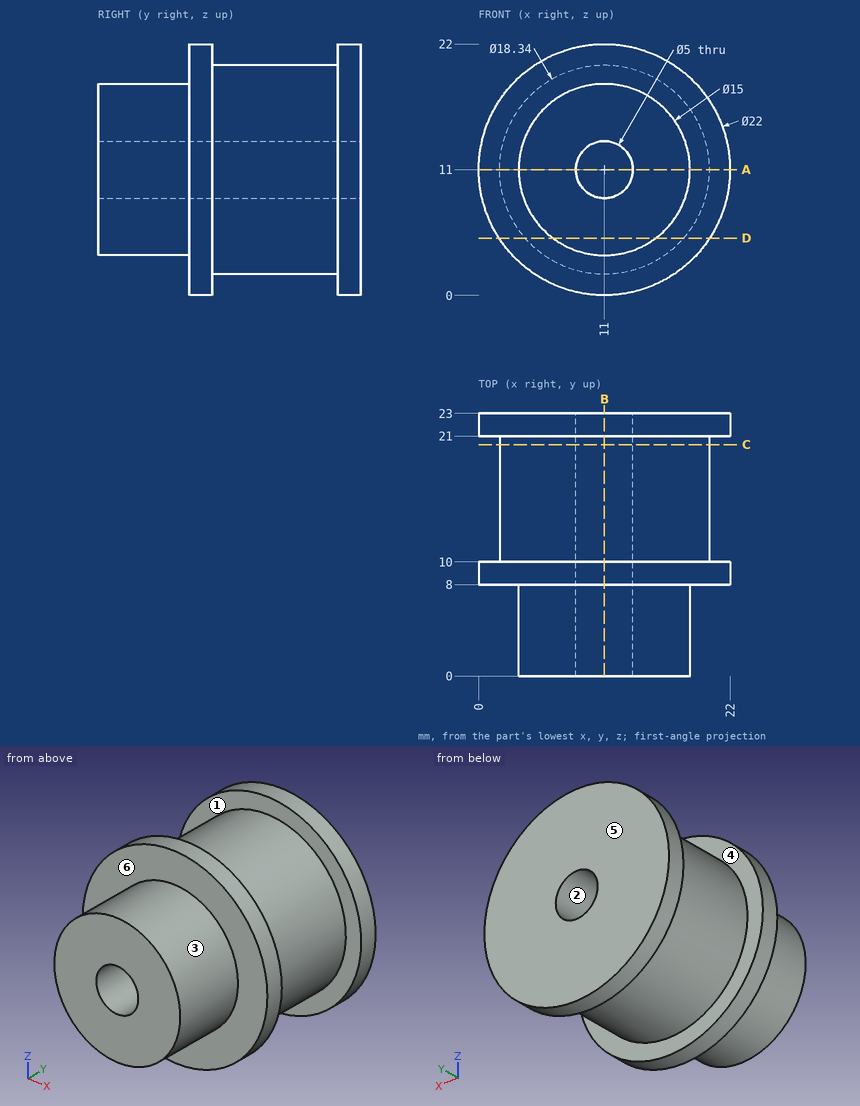
Check sheet for the drawn part. Datum: minimum x, y, z corner. Units: mm. A direction names the side the tool comes from. Round coordinates to 2 decimals unless told otherwise and drop trailing zeros. Order: outer loops, then holes, each group sorted by start corner. A loop starts at its lowest first (then second) coordinate and runs counter-clockwise, first axis right, second up. Notation, with made-up numbers: (89.5, 39.25) -> (123.5, 39.25) arc R9 ccw to (123.5, 56.25) -> close; hole circle Ø9 at (53, 13). An arc over 180 degrees is marked (long way). Put each result on its own line as item: value. Start each with the question number.
(1) Section check B-B (x = 11). Enter the section's corners in (y, z), then the cut area to 3 significant figures.
(2) Draft check along Z on the marked faces 1, 2 and 3. Enter one of: +Z half, -Z half, draft (parallel to the pull), parting line (faces both ways), or undercut.
(3) Section check D-D (z = 5). Enter the section's corners in (x, y).
(4) Depth check by flat-ended pin: pin 1 Ø3 at (x, z) = (3, 6.5) entering from -Y; pin 2 Ø4 at (x, y) = (11, 13.5) entering from +Z; pin 3 Ø5 at (x, y) = (9.5, 2.5) entering from +Z. Enter the tip coordinate at first touch or a pass-through.
(5) Section check A-A (z = 11). Enter the section's corners in (x, y), then the cut area to 3 significant figures.
(6) Section check C-C (y = 20.25). Enter the section's corners in (x, z), then the cut area to 3 significant figures.
(7) Material ranges on line 1 along Y through (x, z) = (11, 20.75); line 2 along X through (y, z) = (14.25, 11); line 3 along X through (y, z) = (6, 11), recorded low to high.
(8) Tool access check on the marked faces 4, 5 and 6. Record the directions out of +Z, -Z, +X, -X, +Y, -Y that give a thin tool (end or side, any length) a straight path to the whole face; none if there is none.
Completed:
1. outline: (0, 3.5) -> (8, 3.5) -> (8, 0) -> (10, 0) -> (10, 1.83) -> (21, 1.83) -> (21, 0) -> (23, 0) -> (23, 8.5) -> (0, 8.5) -> close; (0, 13.5) -> (23, 13.5) -> (23, 22) -> (21, 22) -> (21, 20.17) -> (10, 20.17) -> (10, 22) -> (8, 22) -> (8, 18.5) -> (0, 18.5) -> close
1. area: 295 mm2
2. face 1: draft
2. face 2: undercut
2. face 3: parting line
3. outline: (1.78, 8) -> (6.5, 8) -> (6.5, 0) -> (15.5, 0) -> (15.5, 8) -> (20.22, 8) -> (20.22, 10) -> (17.93, 10) -> (17.93, 21) -> (20.22, 21) -> (20.22, 23) -> (1.78, 23) -> (1.78, 21) -> (4.07, 21) -> (4.07, 10) -> (1.78, 10) -> close
4. pin 1: stops at y = 8
4. pin 2: stops at z = 20.17
4. pin 3: stops at z = 18.5
5. outline: (0, 8) -> (3.5, 8) -> (3.5, 0) -> (8.5, 0) -> (8.5, 23) -> (0, 23) -> (0, 21) -> (1.83, 21) -> (1.83, 10) -> (0, 10) -> close; (13.5, 0) -> (18.5, 0) -> (18.5, 8) -> (22, 8) -> (22, 10) -> (20.17, 10) -> (20.17, 21) -> (22, 21) -> (22, 23) -> (13.5, 23) -> close
5. area: 295 mm2
6. outline: circle Ø18.34 at (11, 11); hole circle Ø5 at (11, 11)
6. area: 245 mm2
7. line 1: y = 8 to 10, 21 to 23
7. line 2: x = 1.83 to 8.5, 13.5 to 20.17
7. line 3: x = 3.5 to 8.5, 13.5 to 18.5
8. face 4: none
8. face 5: +Z, -Z, +X, -X, +Y
8. face 6: -Y
